Could you check a few things on this model? Use its own coordinates, in mm. A direction names the side the tool comes from. Coordinates: 2 decimals unless noted, no trailing zeros. Order: outer loops, then holes, each group sorted by start corner. A loop starts at its lowest first (then second) coordinate and runs counter-clockwise, first axis right, second up. Notation, with made-up numbers: M 68,38 L 118,38 A11 ccw 118,58 Z; hole C 24,-25.5 d11. An arc over 180 degrees is marked long. Write item = value, one per line. Start each with the question number.
from build123d import *

# Parameters (mm, degrees)
F1_DEPTH = 5.842


with BuildPart() as f1:
    # F0 (on Front) → F1 (new body)
    with BuildSketch(Plane.XZ):
        Polygon((23.578767, 80), (-21.421233, 80), (-21.421233, 0), (0.725202, 0), (23.578767, 0), align=None)
        with BuildLine():
            ThreePointArc((-2, 10), (0, 12), (2, 10))
            Line((2, 10), (-2, 10))
        make_face(mode=Mode.SUBTRACT)
    extrude(amount=F1_DEPTH)


solid = f1.part
(1) Please list where this line runs through material, in increasing order: probe 1 along Z at (x, y) = (-0.5, -4.45). Write a range as from..to.
(2) Thinking about a two-plate mould opening in Z: for faces 1 (the flat face through (1, -5.842, 41)), 2 (the cylindrical face through (0, -3, 12)), 3 (the flat face through (1, -3, 80)), which applies, released by +Z, released by -Z, zero draft, split by the parting line, or undercut?
(3) For faces 4 (the flat face through (1, -3, 0)), 5 (the flat face through (0, -3, 10)), which set-ups out of +Z, -Z, +X, -X, +Y, -Y let a thin tool reach every point of the face, with its end or its side?
(4) Will this pin go through, and if not, where does the flat tip stop? P1, Ø1.5, axis at x = -7.5, y = -3.5, coming from the -Z side.
(5) Imagine slicing it at A-A on x = 0. List the corners of the cut face in (y, z) for me, plus the area to 3 significant figures.
Response:
q1.probe_1 = 0..10, 11.94..80
q2.face_1 = zero draft
q2.face_2 = undercut
q2.face_3 = released by +Z
q3.face_4 = -Z, +X, -X, +Y, -Y
q3.face_5 = +Y, -Y
q4.P1 = 0
q5.outline = M -5.84,0 L 0,0 L 0,10 L -5.84,10 Z; M -5.84,12 L 0,12 L 0,80 L -5.84,80 Z
q5.area = 456 mm2
